The listing builds one solid part. Answer for the finished solid, in the listing's coordinates (mm). Face numbers are marked on the shaded views. A direction names the side the tool comes from. Give positions to 0.01 mm unless a question says otherwise; leave off trailing zeros. Order: outer loops, then holes, each group sorted by start corner. A loop starts at its lowest first (then second) coordinate and runs counter-clockwise, first axis right, second up. Notation, with made-up numbers: (72, -33.5) - (76, -33.5) arc R14 cw to (76, -19.5) - close; hole circle Ø5 at (51.25, -32). An arc over 180 degrees is marked (long way). Answer as a JSON object with one key per item and string values. Group by question number.
Q1. Consider line 1 (Z direction, x = 342, y = 128.5); line 2 (Y direction, x = 284.5, z = 1312); line 3 (Z direction, x = 288.5, y = 90.5). Determine where each line is inside the solid, lowest interval first.
Q2. A cutting plane is placed at A-A, the plane z = 1393. Give the vertices of the cut face in (x, y), and give its area (3 significant figures).
Q3. A cutting plane is placed at B-B, the plane x = 242.5. Count the separate pieces of the cut face and the enclosed holes in it, and give its area (3 significant figures).
Q4. For the marked faces 1 and 2, determine the directions among +Z, -Z, +X, -X, +Y, -Y from which every point of the face is accessible in a straight line to the end or side of a thin tool.
Q5. Given pin 1 (6 mm diameter, centred on x = 348.5, z = 1233, fed in from +Y); pin 2 (4 mm diameter, centred on x = 242.5, z = 499.5, fed in from -Y); pin 3 (10 mm diameter, centred on x = 244, z = 659, fed in from -Y), each flat-ended and moving along its own axis, determine where each tip first touches the part or whether it passes through.
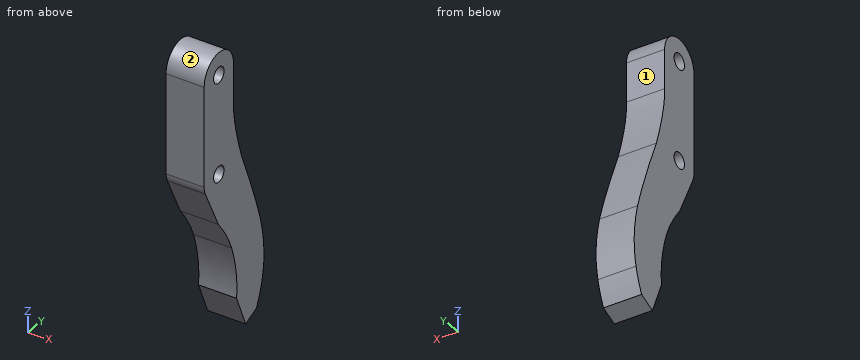
Autodesk Inventor part; units mm, degrees
ref_plane "YZ Plane" through (0, 0, 0) normal (1, 0, 0) x (0, 1, 0)
ref_plane "XZ Plane" through (0, 0, 0) normal (0, 1, 0) x (-1, 0, 0)
ref_plane "XY Plane" through (0, 0, 0) normal (0, 0, 1) x (1, 0, 0)
ref_plane "Work Plane1" through (215.9, 467.0605, 68.1432) normal (1, 0, 0) x (0, 1, 0)
sketch "Sketch1" plane through (215.9, 467.0605, 68.1432) normal (1, 0, 0) x (0, 1, 0)
  line L0 (-213.126, 1464.2722) -> (-213.126, 1242.4656)
  spline S0 degree 2 poles (-213.126, 1242.4656) (-217.9428, 1125.9893) (-141.0804, 895.2277) knots 0 0 0 1 1 1
  spline S1 degree 2 poles (-141.0804, 895.2277) (-30.9453, 631.5803) (21.2303, 454.393) knots 0 0 0 1 1 1
  spline S2 degree 2 poles (21.2303, 454.393) (72.7957, 260.8739) (34.9413, 105.2911) knots 0 0 0 1 1 1
  spline S3 degree 2 poles (34.9413, 105.2911) (19.2909, 39.5013) (-13.3827, -28.1704) knots 0 0 0 1 1 1
  line L1 (-13.3827, -28.1704) -> (-107.2389, -68.1432)
  line L2 (-107.2389, -68.1432) -> (-185.683, 119.1347)
  spline S4 degree 2 poles (-185.683, 119.1347) (-171.2271, 262.5707) (-229.4608, 427.494) knots 0 0 0 1 1 1
  spline S5 degree 2 poles (-229.4608, 427.494) (-265.2584, 523.1386) (-344.3827, 623.2364) knots 0 0 0 1 1 1
  line L3 (-344.3827, 623.2364) -> (-467.0605, 875.6763)
  line L4 (-467.0605, 1464.2722) -> (-467.0605, 875.6763)
  arc A0 (-213.126, 1464.2722) -> (-467.0605, 1464.2722) centre (-340.0933, 1464.2722) ccw
  circle A1 centre (-340.0933, 1464.2722) radius 45
  circle A2 centre (-340.0933, 904.6692) radius 45
  point P0 (-467.0605, -68.1432)
  point P1 (-203.4806, 1128.5151)
  point P2 (-36.7776, 629.4713)
  point P3 (50.7616, 260.3303)
  point P4 (15.6727, 40.7996)
  point P5 (-188.3614, 260.3302)
  point P6 (-272.8905, 518.7472)
  dimension "d0" = 90
  dimension "d1" = 90
  dimension "d5" = 126.9673
extrude "Extrusion1" add sketch "Sketch1" along normal blind 215.9
fillet "Fillet1" radius 100 1 edges at (323.85, 0, 943.8196)
properties part number "Final Gripper 1"
Reply:
{
 "1": {"line 1": "z = 683.94 to 927.84, 1017.79 to 1487.44, 1577.39 to 1659.37", "line 2": "y = 0 to 253.93", "line 3": "z = 757.59 to 946.45, 999.18 to 1506.05, 1558.78 to 1654.03"},
 "2": {"outline": "(215.9, 0) - (431.8, 0) - (431.8, 253.93) - (215.9, 253.93) - close", "area": "54,800 mm^2"},
 "3": {"separate pieces": "1", "enclosed holes": "2", "area": "410,000 mm^2"},
 "4": {"face 1": "+Z, +X, -X, +Y", "face 2": "+Z, +X, -X"},
 "5": {"pin 1": "stops at y = 258.45", "pin 2": "stops at y = 235.37", "pin 3": "stops at y = 143.57"}
}
